from build123d import *

# Parameters (mm, degrees)
F1_DEPTH = 6.96


with BuildPart() as f1:
    # F0 (on Front) → F1 (new body)
    with BuildSketch(Plane.XZ):
        with BuildLine():
            Line((7.764825, -37.187766), (7.764825, -37.751798))
            Line((7.764825, -37.751798), (8.341329, -37.187766))
            Line((8.341329, -37.187766), (37.133072, -7.022527))
            ThreePointArc((37.133072, -7.022527), (40.255881, 0.371149), (37.133072, 7.764825))
            Line((37.133072, 7.764825), (7.861621, 37.010901))
            ThreePointArc((7.861621, 37.010901), (0.040821, 40.394728), (-7.689789, 36.809638))
            Line((-7.689789, 36.809638), (-37.264177, 7.930262))
            ThreePointArc((-37.264177, 7.930262), (-40.565071, 0.5208), (-37.264177, -6.888662))
            Line((-37.264177, -6.888662), (-7.694786, -37.053901))
            ThreePointArc((-7.694786, -37.053901), (-1.330862, -41.685065), (6.172718, -39.309461))
            ThreePointArc((6.172718, -39.309461), (7.049861, -38.309462), (7.764825, -37.187766))
        make_face()
        with BuildLine():
            ThreePointArc((-7.764906, -7.79142), (-8.124877, -7.415279), (-8.466647, -7.022527))
            ThreePointArc((-8.466647, -7.022527), (0, 11), (8.466647, -7.022527))
            ThreePointArc((8.466647, -7.022527), (8.124839, -7.415322), (7.764825, -7.791501))
            ThreePointArc((7.764825, -7.791501), (-5.7e-05, -11), (-7.764906, -7.79142))
        make_face(mode=Mode.SUBTRACT)
    extrude(amount=F1_DEPTH)


solid = f1.part
Could you check a few things on this model? Use its own coordinates, in mm. A direction names the side the tool comes from. Round coordinates to 2 decimals unless told otherwise and drop trailing zeros. Order: outer loops, then holes, each group sorted by start corner. A loop starts at its lowest first (then second) coordinate and runs counter-clockwise, first axis right, second up.
(1) Imagine slicing it at C-C (x = 0). Write out the boundary of the cut face in (y, z).
Response values:
outline: (-6.96, -41.8) - (0, -41.8) - (0, -11) - (-6.96, -11) - close; (-6.96, 11) - (0, 11) - (0, 40.39) - (-6.96, 40.39) - close
(2) Imagine slicing it at B-B (z = 0). Write out the boundary of the cut face in (x, y), plus the area to 3 significant figures.
Response values:
outline: (-40.55, -6.96) - (-11, -6.96) - (-11, 0) - (-40.55, 0) - close; (11, -6.96) - (40.25, -6.96) - (40.25, 0) - (11, 0) - close
area: 409 mm2
(3) Please list where these lines run through material, in increasing order: line 1 along Z through (x, y) = (0, -2.5); line 2 along X through (y, z) = (-2.75, 0); line 3 along Z through (x, y) = (-1, -3.5).
Response values:
line 1: z = -41.8 to -11, 11 to 40.39
line 2: x = -40.55 to -11, 11 to 40.25
line 3: z = -41.73 to -10.95, 10.95 to 40.33
(4) Imagine slicing it at D-D (x = 26). Write out the boundary of the cut face in (y, z), plus the area to 3 significant figures.
Response values:
outline: (-6.96, -18.69) - (0, -18.69) - (0, 18.89) - (-6.96, 18.89) - close
area: 262 mm2
(5) Which directions (+Z, -Z, +X, -X, +Y, -Y) give clear straight access to the entire face, cutting with the end or side of a thin tool? Please do faces 1 (the flat face through (22.702, -3.431, 22.183)), 2 (the cylindrical face through (0, -3, -11)).
Response values:
face 1: +Z, +X, +Y, -Y
face 2: +Y, -Y
(6) Imagine slicing it at A-A (y = -4.75). Write out the boundary of the cut face in (x, z).
Response values:
outline: (-37.26, -6.89) - (-7.69, -37.05) arc R8.73 ccw to (6.17, -39.31) arc R8.73 ccw to (7.76, -37.19) - (7.76, -37.75) - (8.34, -37.19) - (37.13, -7.02) arc R10.31 ccw to (37.13, 7.76) - (7.86, 37.01) arc R10.42 ccw to (-7.69, 36.81) - (-37.26, 7.93) arc R9.97 ccw to start; hole (-8.47, -7.02) arc R11 ccw to (-7.76, -7.79) arc R11 ccw to (7.76, -7.79) arc R11 ccw to (8.47, -7.02) arc R11 ccw (long way) to start
(7) I'm going to push flat-ended pins straight in: pin 1 (1.5 mm diameter, centred on x = 9.5, z = -3, fed in from +Y); pin 2 (1.5 mm diameter, centred on y = -5, z = -11, fed in from +X); pin 3 (1 mm diameter, centred on x = -15.5, y = -4.5, fed in from -Z); pin 4 (2 mm diameter, centred on y = -4.5, z = 2.5, fed in from +X). Where does each tip first touch, or does it pass through?
Response values:
pin 1: passes through
pin 2: stops at x = 34.05
pin 3: stops at z = -29.6
pin 4: stops at x = 40.19
(8) If we mould it in two halves opening along X, with no side actions, what happens to faces 3 (the cylindrical face through (0.164, -3.431, 40.396)), 4 (the flat face through (8, 0, 9)), 5 (the cylindrical face through (0, -3, 11))? For each: released by +X, released by -X, zero draft, split by the parting line, or undercut.
Response values:
face 3: split by the parting line
face 4: zero draft
face 5: undercut
